from build123d import *

# Parameters (mm, degrees)
ESQUISSE2_R        = 2.5
ESQUISSE3_R        = 4
BOSS_EXTRU_1_DEPTH = 45


with BuildPart() as part:
    # Balayage1: sweep along a path in Esquisse1
    with BuildLine(Plane.XY) as balayage1_path:
        Line((0, 0), (30, 0))
        ThreePointArc((30, 0), (37.071067812, 2.928932188), (40, 10))
        Line((40, 10), (40, 20))
        ThreePointArc((40, 20), (42.928932188, 27.071067812), (50, 30))
        Line((50, 30), (100, 30))
    # Esquisse2 → Balayage1 (sweep)
    with BuildSketch(Plane(origin=(100, 0, 0), x_dir=(0, 0, -1), z_dir=(1, 0, 0))):
        with Locations((0, 30)):
            Circle(ESQUISSE2_R)
    sweep(path=balayage1_path.line)

    # Esquisse3 → Boss.-Extru.1 (add)
    with BuildSketch(Plane(origin=(100, 0, 0), x_dir=(0, 0, -1), z_dir=(1, 0, 0))):
        with Locations((0, 30)):
            Circle(ESQUISSE3_R)
    extrude(amount=-BOSS_EXTRU_1_DEPTH)


solid = part.part
Input: part model. Units: mm. Frame: model coordinates. A direction names the side the tool comes from. Round coordinates to 2 decimals unless told otherwise and drop trailing zeros. Order: outer loops, then holes, each group sorted by start corner. A loop starts at its lowest first (then second) coordinate and runs counter-clockwise, first axis right, second up. Notation, with made-up numbers: (-35.75, -34.75) - (-19.75, -34.75) arc R6 ccw to (-19.75, -23.75) - close; hole circle Ø8 at (-21, -3.75). An arc over 180 degrees is marked (long way). Answer as a JSON object with one key per item and string values. Group by question number.
(1) Cut plane C-C (x = 63.5). Return loops of the section in (y, z).
(2) Reachability of faces 1 (the face through (100, 30, 0)), 2 (the face through (77.815, 33.966, 0.521)), 3 (the face through (55, 32, -2)) from +Z, -Z, +X, -X, +Y, -Y: full face, straight path, thin tool, end or side. Return the list, or none.
(3) Material intervals for probe 1 along Y at (x, z) = (54.5, -0.25); probe 2 along X at (y, z) = (30.5, -2.75); probe 3 along Y at (x, z) = (75.5, 1.5), sorted ascending. Write a range as from..to.
(4) Pin query (flat end, axial travel): P1, Ø3, axis at x = 59.5, z = 2, coming from the +Y side; P2, Ø1, axis at x = 11, z = -2.5, coming from the +Y side; P3, Ø2, axis at x = 81, y = 27.5, coming from the -Z side. Return the tip coordinate at first contact, or that it passes through.
(5) Cut plane A-A (z = 0). Return loops of the section in (x, y).
(6) Cut plane B-B (x = 19.5). Return loops of the section in (y, z), then the cut area to 3 significant figures.
(7) Draft query along X for faces 4 (the face through (42.44, 15.07, 0.54)), 5 (the face through (52.54, 32.11, -1.34)), 6 (the face through (0, 0, 0)), 7 (the face through (15.21, -2.44, 0.54)). Return one class per face: released by +X, released by -X, zero draft, split by the parting line, or undercut.
Here are the results:
{
 "1": {"outline": "circle Ø8 at (30, 0)"},
 "2": {"face 1": "+Z, -Z, +X, +Y, -Y", "face 2": "+X", "face 3": "none"},
 "3": {"probe 1": "y = 27.51..32.49", "probe 2": "x = 55..100", "probe 3": "y = 26.29..33.71"},
 "4": {"P1": "stops at y = 33.97", "P2": "stops at y = 1.5", "P3": "stops at z = -3.71"},
 "5": {"outline": "(0, -2.5) - (30, -2.5) arc R12.5 ccw to (42.5, 10) - (42.5, 20) arc R7.5 cw to (50, 27.5) - (55, 27.5) - (55, 26) - (100, 26) - (100, 34) - (55, 34) - (55, 32.5) - (50, 32.5) arc R12.5 ccw to (37.5, 20) - (37.5, 10) arc R7.5 cw to (30, 2.5) - (0, 2.5) - close"},
 "6": {"outline": "circle Ø5 at (0, 0)", "area": "19.6 mm^2"},
 "7": {"face 4": "split by the parting line", "face 5": "undercut", "face 6": "released by -X", "face 7": "zero draft"}
}
